Here's the drawing with two shaded views (mm, measured from the low corner). I have some questions. Round coordinates to 2 decimals unless told otherwise and drop trailing zeros. Loops run counter-clockwise (first coordinate to the right, second up) from the corner with the lowest first, then second, coordinate; pieces in that order, holes last.
(1) If I drill on line 1 along X through (y, z) = (1.4, 21.5); line 2 along Z through (x, y) = (24, 3) (1 decimal), over which ranges is the centre line in solid material (lowest first)?
(2) I want a section at B-B on y = 1.55. Write out the boundary of the cut face in (x, z) (1 decimal), plus the area to 3 significant figures.
(3) I want a section at A-A on z = 18. Write out the boundary of the cut face in (x, y) (1 decimal), plus the area to 3 significant figures.
(4) I want a section at C-C on x = 25. Write out the boundary of the cut face in (y, z) (1 decimal).
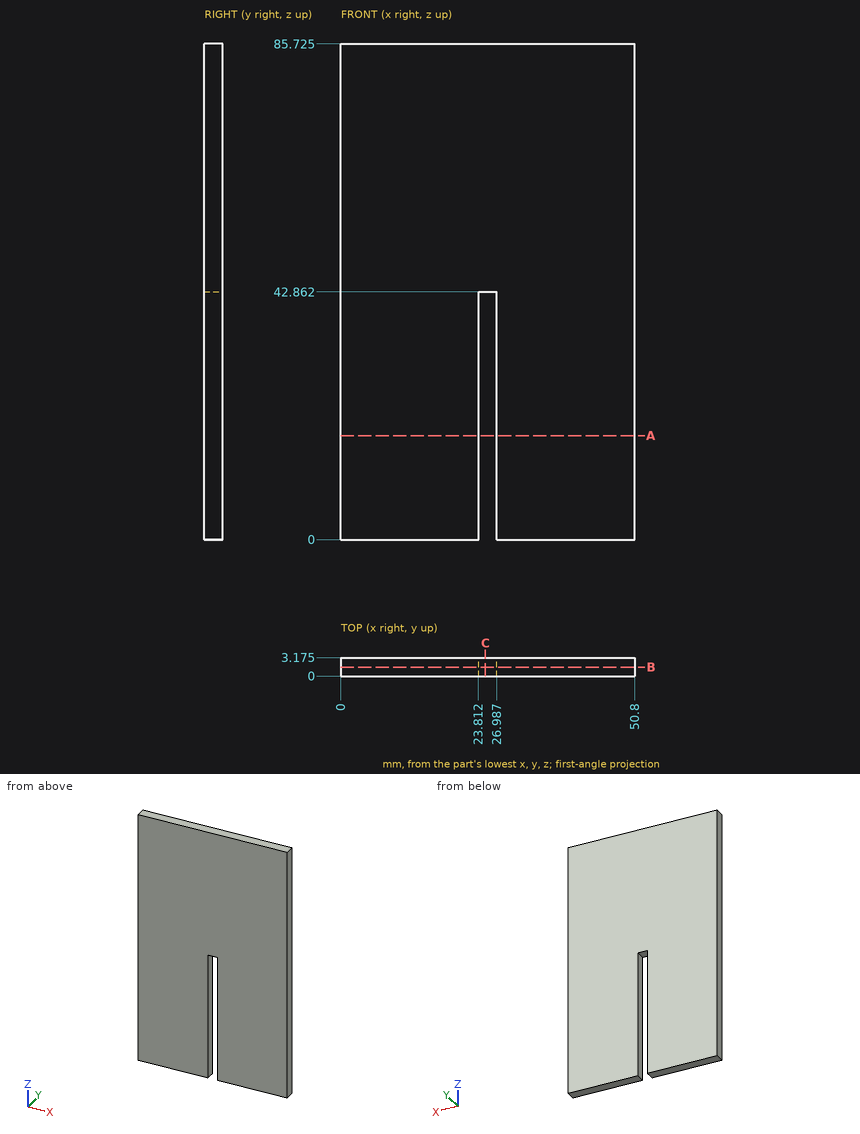
Filled sheet:
1. line 1: x = 0 to 23.81, 26.99 to 50.8
1. line 2: z = 42.9 to 85.7
2. outline: (0, 0) - (23.8, 0) - (23.8, 42.9) - (27, 42.9) - (27, 0) - (50.8, 0) - (50.8, 85.7) - (0, 85.7) - close
2. area: 4,220 mm2
3. outline: (0, 0) - (23.8, 0) - (23.8, 3.2) - (0, 3.2) - close; (27, 0) - (50.8, 0) - (50.8, 3.2) - (27, 3.2) - close
3. area: 151 mm2
4. outline: (0, 42.9) - (3.2, 42.9) - (3.2, 85.7) - (0, 85.7) - close
